Study the drawing (mm; zero at the part's minimum x, y, z) and answer. Coordinates: 2 decimals unless noted, no trailing zeros. Write each loop counter-clockwise with the first axis right and the second up, starting at its lowest first coordinate (ties: lowest second). Pieces come first, ordered by that corner, then holes. Notation, with made-up numbers: (83.5, 33.5) -> (107.5, 33.5) arc R19 ccw to (107.5, 60.5) -> close; hole circle Ø8 at (39, 28.5). An arc over 180 degrees is marked (long way). Write item = value, one per line. Start each with the question number.
1) Flat-ended cylindrical pins translate along their axes: pin 1 Ø2.5 at (x, y) = (83.5, 85) entering from +Z; pin 2 Ø0.9 at (x, z) = (1.5, 33) entering from -Y. Find the tip coordinate at first contact, or state that the pin passes through.
2) Section B-B (y = 10) is taken. Determine the outline of the cut face in (x, z).
3) Section D-D (z = 45) is taken. Determine the outline of the cut face in (x, y), plus the area to 3 significant figures.
4) Section A-A (z = 13.5) is taken. Count the separate pieces of the cut face and the enclosed holes in it, plus the area to 3 significant figures.
5) Section C-C (x = 66) is taken. Determine the outline of the cut face in (y, z), plus the area to 3 significant figures.
6) For a pull along X with two mould halves and no side action, classify the marked faces 1, 2, 3 and 4 as released by +X, released by -X, zero draft, split by the parting line, or undercut.
7) Find the intervals of material crossed by line 1 along Z through (x, y) = (83.3, 81.5); line 2 along Z through (x, y) = (1.2, 81.5); line 3 along Z through (x, y) = (0.9, 89.5), in increasing order. Write a range as from..to.
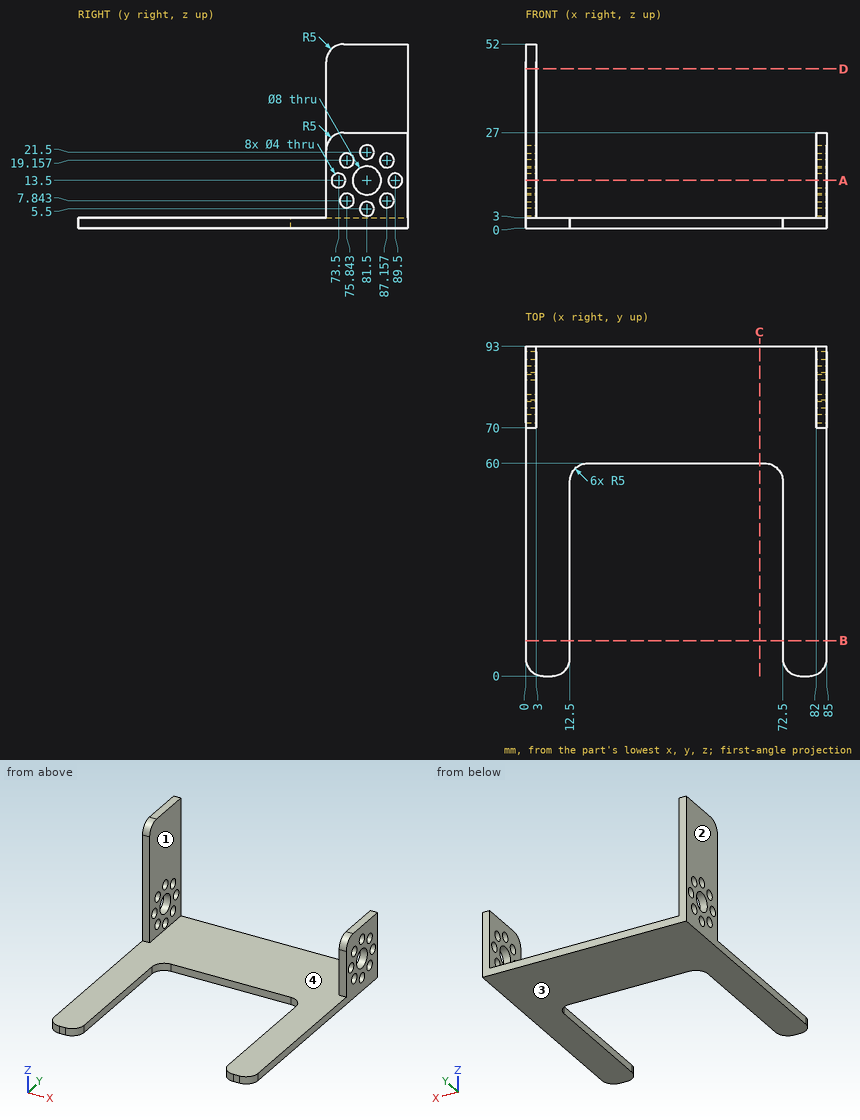
Answer key:
q1.pin_1 = 27
q1.pin_2 = 70
q2.outline = (0, 0) -> (12.5, 0) -> (12.5, 3) -> (0, 3) -> close; (72.5, 0) -> (85, 0) -> (85, 3) -> (72.5, 3) -> close
q3.outline = (0, 70) -> (3, 70) -> (3, 93) -> (0, 93) -> close
q3.area = 69.0 mm^2
q4.separate_pieces = 8
q4.enclosed_holes = 0
q4.area = 42.0 mm^2
q5.outline = (60, 0) -> (93, 0) -> (93, 3) -> (60, 3) -> close
q5.area = 99.0 mm^2
q6.face_1 = undercut
q6.face_2 = released by -X
q6.face_3 = zero draft
q6.face_4 = undercut
q7.line_1 = 0..3.5, 7.5..9.5, 17.5..19.5, 23.5..27
q7.line_2 = 0..3.5, 7.5..9.5, 17.5..19.5, 23.5..52
q7.line_3 = 0..11.5, 15.5..52
